Autodesk Inventor part; units mm, degrees
ref_plane "YZ Plane" through (0, 0, 0) normal (1, 0, 0) x (0, 1, 0)
ref_plane "XZ Plane" through (0, 0, 0) normal (0, 1, 0) x (-1, 0, 0)
ref_plane "XY Plane" through (0, 0, 0) normal (0, 0, 1) x (1, 0, 0)
sketch "Sketch1" plane through (0, 0, 0) normal (0, 0, 1) x (1, 0, 0)
  circle A0 centre (0, 0) radius 3.175
  circle A1 centre (0, 0) radius 6.35
  dimension "d0" = 12.7
  dimension "d1" = 6.35
extrude "Extrusion1" add sketch "Sketch1" along normal blind 63.5
sketch "Sketch2" plane through (0, 0, 0) normal (0, 0, -1) x (-1, 0, 0)
  circle A0 centre (0, 0) radius 6.35
  arc A1 (-1.575, 6.1516) -> (1.575, 6.1516) centre (0, 6.35) ccw
  line L0 (0, 6.35) -> (0, 0) construction
  arc A2 (1.575, 6.1516) -> (-1.575, 6.1516) centre (0, 0) ccw
  dimension "d4" = 1.5875
extrude "Extrusion2" cut sketch "Sketch2" against normal through all contours A1 A0 picked at (0, 5.8061)
pattern_circular "Circular Pattern1" count 6 over 360 about axis through (0, 0, 0) along (0, 0, 1) of "Extrusion2"
properties part number "HopperPlateOffset" material "Aluminum-6061"
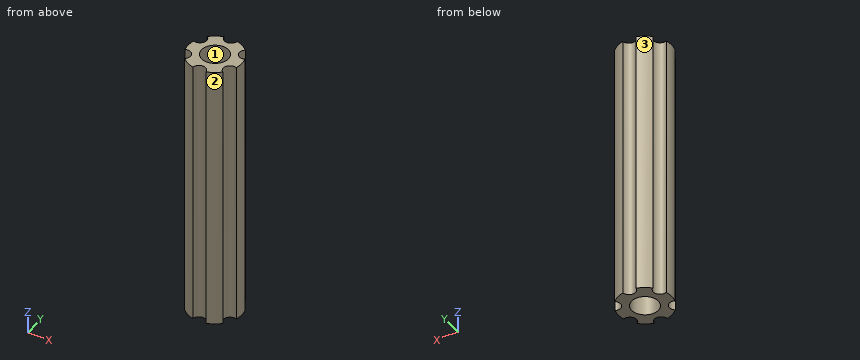
Model file for the job. Use its own axes, mm. Face numbers are marked on the shaded views. Give positions to 0.01 mm unless a question says otherwise; leave off trailing zeros. Order: outer loops, then holes, each group sorted by start corner. A loop starts at its lowest first (then second) coordinate and runs counter-clockwise, first axis right, second up. Notation, with made-up numbers: (-38.75, 49) - (-1.75, 49) arc R26 ccw to (-1.75, 86) - close; hole circle Ø7 at (-33, -33). An arc over 180 degrees is marked (long way). Return JSON: item names as keys, results as strings.
1) Cut at C-C, the plane z = 5.5. Give the cut face in (x, y) (3 decimals).
Geometry says:
{"outline": "(-6.115, -1.712) arc R1.587 cw to (-4.54, -4.44) arc R6.35 ccw to (-1.575, -6.152) arc R1.587 cw to (1.575, -6.152) arc R6.35 ccw to (4.54, -4.44) arc R1.587 cw to (6.115, -1.712) arc R6.35 ccw to (6.115, 1.712) arc R1.587 cw to (4.54, 4.44) arc R6.35 ccw to (1.575, 6.152) arc R1.587 cw to (-1.575, 6.152) arc R6.35 ccw to (-4.54, 4.44) arc R1.587 cw to (-6.115, 1.712) arc R6.35 ccw to start; hole circle Ø6.35 at (0, 0)"}
2) Probe line 1 (Y direction, x = 0, z = 32) (3 decimals); line 2 (Y direction, x = 4.25, z = 38); line 3 (Y direction, x = -1, z = 21.5). List the from-to ranges inside material, lowest first. Write a range as from..to.
Geometry says:
{"line 1": "-4.763..-3.175, 3.175..4.763", "line 2": "-4.72..-4.15, -2.2..2.2, 4.15..4.72", "line 3": "-5.12..-3.01, 3.01..5.12"}
3) Flat gauge pins, fed straight in: P1, Ø1, axis at y = -4.5, z = 13, coming from the +X side; P2, Ø2, axis at x = -3.5, z = 31, coming from the -Y side; P3, Ø4, axis at y = 3.5, z = 45.5, coming from the -X side. Where does each tip first touch, or does it go through?
Geometry says:
{"P1": "x = 4.54", "P2": "y = -5.84", "P3": "x = -6.17"}
4) Cut at B-B, the plane y = 0. Give the cut face in (x, z) (3 decimals), plus the area to 3 significant figures.
Geometry says:
{"outline": "(-6.35, 0) - (-3.175, 0) - (-3.175, 63.5) - (-6.35, 63.5) - close; (3.175, 0) - (6.35, 0) - (6.35, 63.5) - (3.175, 63.5) - close", "area": "403 mm²"}
5) Cut at A-A, the plane x = 0. Give the cut face in (y, z) (3 decimals), plus the area to 3 significant figures.
Geometry says:
{"outline": "(-4.763, 0) - (-3.175, 0) - (-3.175, 63.5) - (-4.763, 63.5) - close; (3.175, 0) - (4.763, 0) - (4.763, 63.5) - (3.175, 63.5) - close", "area": "202 mm²"}
6) Pull direction X, two halves, no side cores. Call the marked faces 1, 2 and 3: pulls with the +X half, pulls with the -X half, needs draft (parallel to the pull), parting line crosses it, or undercut.
Geometry says:
{"face 1": "undercut", "face 2": "pulls with the +X half", "face 3": "pulls with the -X half"}
